The listing builds one solid part. Answer for the finished solid, in the listing's coordinates (mm). Face numbers are marked on the shaded views. A direction names the side the tool comes from. Round coordinates to 2 decimals unless told otherwise and drop trailing zeros. Loops run counter-clockwise (first coordinate to the right, second up) from the corner with the lowest first, then second, coordinate; pieces in that order, holes last. Notation, with made-up numbers: M -40,0.5 L -4,0.5 A15 ccw -4,7.5 Z; hole C 44,58 d10. An arc over 180 degrees is marked long. Answer as a JSON object with one key per item and string values.
```python
from build123d import *


with BuildPart() as part:
    # Sketch1 → Revolve1 (O-Rings : 2-141 & 2-144) (revolve)
    with BuildSketch(Plane(origin=(0, 0, 0), x_dir=(0, 0, -1), z_dir=(1, 0, 0)), mode=Mode.PRIVATE) as revolve1_o_rings_2_141_2_144_sk:
        Polygon((0, 28.4734), (0, 32.8676), (6.1722, 32.8676), (6.1722, 34.8996), (-3.175, 34.8996), (-3.175, 32.8676), (-6.858, 32.8676), (-6.858, 34.8996), (-9.398, 34.8996), (-9.398, 32.8676), (-13.081, 32.8676), (-13.081, 34.8996), (-30.69336, 34.8996), (-30.69336, 32.512), (-36.40836, 32.512), (-36.40836, 30.48), (-40.09136, 30.48), (-40.09136, 32.512), (-42.63136, 32.512), (-42.63136, 30.48), (-46.31436, 30.48), (-46.31436, 32.512), (-49.48936, 32.512), (-49.48936, 28.4734), align=None)
    revolve(revolve1_o_rings_2_141_2_144_sk.sketch.rotate(Axis((0, 0, 0), (0, 0, 1)), 90), axis=Axis((0, 0, 0), (0, 0, 1)))


solid = part.part
```
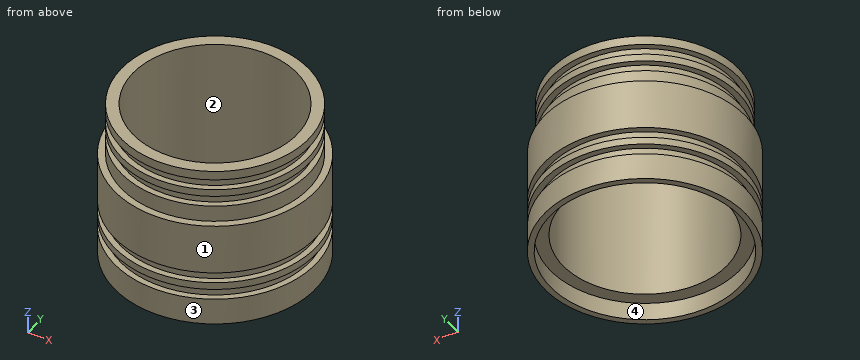
Item 1: Straight lines are drawn through the part: line 1 (Z direction, x = 31, y = -11) (3 decimals); line 2 (Y direction, x = 0, z = -4); line 3 (Y direction, x = 0, z = 38). For each, find the intervals that lie inside material, in ascending order.
Values follow:
{"line 1": "-6.172 to 3.175, 6.858 to 9.398, 13.081 to 30.693", "line 2": "-34.9 to -32.87, 32.87 to 34.9", "line 3": "-30.48 to -28.47, 28.47 to 30.48"}
Item 2: The part is cut by section A-A (z = 44). Give the vertices of the cut face in (x, y).
Values follow:
{"outline": "C 0,0 d60.96; hole C 0,0 d56.95"}
Item 3: The part is cut by section B-B (z = 29.5). Give the vertices of the cut face in (x, y), then the cut area to 3 significant figures.
Values follow:
{"outline": "C 0,0 d69.8; hole C 0,0 d56.95", "area": "1,280 mm^2"}
Item 4: Determine the mould class of the marked faces 1 and 2 for opening direction Y: released by +Y, released by -Y, zero draft, split by the parting line, or undercut.
Values follow:
{"face 1": "split by the parting line", "face 2": "undercut"}
Item 5: Which of the six approach directions +Z, -Z, +X, -X, +Y, -Y give full straight-line access (tool end or side, diameter ignored) to the marked faces 3 and 4?
Values follow:
{"face 3": "+Z, -Z", "face 4": "-Z"}
Item 6: Flat-ended cylindrical pins translate along their axes: P1, Ø3, axis at y = -1.5, z = 6, coming from the +X side; P2, Ø6, axis at y = -9, z = 38.5, coming from the -X side; P3, Ø21, axis at x = 5.5, y = -7, coming from the +Z side; P4, Ø3, axis at x = -11.5, z = 6.5, coming from the -Y side. Find the tip coordinate at first contact, or state that the pin passes through.
Values follow:
{"P1": "x = 34.9", "P2": "x = -31.86", "P3": "through", "P4": "y = -33.42"}
